from build123d import *

# Parameters (mm, degrees)
SKETCH1_W             = 254
SKETCH1_H             = 152.4
BOSS_EXTRUDE1_DEPTH   = 6
SKETCH2_W             = 25.4
SKETCH2_H             = 5.588
SKETCH2_W_2           = 31.75
SKETCH2_H_2           = 2.7432
TABS_TOP_BOTTOM_DEPTH = 6
SKETCH3_W             = 5.588
SKETCH3_H             = 25.4508
TABS_SIDE_DEPTH       = 6


with BuildPart() as part:
    # Sketch1 → Boss-Extrude1 (new body)
    with BuildSketch(Plane(origin=(0, 0, 0), x_dir=(1, 0, 0), z_dir=(0, 1, 0))):
        Rectangle(SKETCH1_W, SKETCH1_H)
    extrude(amount=BOSS_EXTRUDE1_DEPTH)

    # Sketch2 → Tabs - Top/Bottom (add)
    with BuildSketch(Plane(origin=(0, 6, 0), x_dir=(1, 0, 0), z_dir=(0, 1, 0))):
        with Locations((95.25, 78.994)):
            Rectangle(SKETCH2_W, SKETCH2_H)
        with Locations((-95.25, 78.994)):
            Rectangle(SKETCH2_W, SKETCH2_H)
        with Locations((-31.75, 78.994)):
            Rectangle(SKETCH2_W, SKETCH2_H)
        with Locations((31.75, 78.994)):
            Rectangle(SKETCH2_W, SKETCH2_H)
        with Locations((-95.25, -77.5716)):
            Rectangle(SKETCH2_W_2, SKETCH2_H_2)
        with Locations((0, -77.5716)):
            Rectangle(SKETCH2_W_2, SKETCH2_H_2)
        with Locations((95.25, -77.5716)):
            Rectangle(SKETCH2_W_2, SKETCH2_H_2)
    extrude(amount=-TABS_TOP_BOTTOM_DEPTH)

    # Sketch3 → Tabs - Side (add)
    with BuildSketch(Plane(origin=(0, 6, 0), x_dir=(1, 0, 0), z_dir=(0, 1, 0))):
        with Locations((-129.794, -38.1)):
            Rectangle(SKETCH3_W, SKETCH3_H)
        with Locations((-129.794, 0)):
            Rectangle(SKETCH3_W, SKETCH3_H)
        with Locations((-129.794, 38.1)):
            Rectangle(SKETCH3_W, SKETCH3_H)
        with Locations((129.794, -38.1)):
            Rectangle(SKETCH3_W, SKETCH3_H)
        with Locations((129.794, 38.1)):
            Rectangle(SKETCH3_W, SKETCH3_H)
        with Locations((129.794, 0)):
            Rectangle(SKETCH3_W, SKETCH3_H)
    extrude(amount=-TABS_SIDE_DEPTH)


solid = part.part
Work out the finished part from the listing and answer in its coordinate system (mm). A direction names the side the tool comes from. Round coordinates to 2 decimals unless told otherwise and drop trailing zeros. Write each loop counter-clockwise with the first axis right and the second up, starting at its lowest first coordinate (ties: lowest second). Pieces come first, ordered by that corner, then holes. Notation, with made-up numbers: (-39.75, 85.5) -> (-9.75, 85.5) arc R20 ccw to (-9.75, 108.5) -> close; hole circle Ø1 at (58.25, -36.5). An arc over 180 degrees is marked (long way). Answer as CSV lines item,"result". Start each with the question number.
(1) The part is cut by section A-A, the plane x = -22. Give the vertices of the cut face in (y, z), then the cut area to 3 significant figures.
(2) Each of these flat-tipped pins is pushed along its axis until it touches: pin 1 (3 mm diameter, centred on y = 2, z = 78, fed in from +X) (3 decimals); pin 2 (3 mm diameter, centred on y = 2.5, z = -80, fed in from -X); pin 3 (3 mm diameter, centred on y = 2, z = -79.5, fed in from +X); pin 4 (6 mm diameter, centred on x = -91, z = 0.5, fed in from -Y). Where does it stop, or does it pass through?
(3) The part is cut by section B-B, the plane z = -54.5. Give the vertices of the cut face in (x, y).
(4) A tool of negligible diameter and unlimited length cuts with its end or side. For faces 1 (the flat face through (47, 3, 76.2)), 2 (the flat face through (-119, 3, 76.2)), 3 (the flat face through (-130, 3, 12.725)), from which of +Z, -Z, +X, -X, +Y, -Y can it reach the whole face along a straight path? Write none if from no direction.
(5) The mould has two halves that part along Z. Classify faces 4 (the flat face through (130, 3, 25.375)), 5 (the flat face through (0, 3, -76.2)), 6 (the flat face through (-44.45, 3, -79)): +Z half, -Z half, draft (parallel to the pull), parting line (faces both ways), or undercut.
(6) Find the intervals of material crossed by probe 1 along Z at (x, y) = (-119, 1.15); probe 2 along X at (y, z) = (5.6, 68); probe 3 along Z at (x, y) = (-1.5, 2.5), in increasing order.
Output values:
1,outline,"(0, -81.79) -> (6, -81.79) -> (6, 76.2) -> (0, 76.2) -> close"
1,area,"948 mm²"
2,pin 1,"stops at x = 111.125"
2,pin 2,"stops at x = -107.95"
2,pin 3,"stops at x = 107.95"
2,pin 4,"stops at y = 0"
3,outline,"(-127, 0) -> (127, 0) -> (127, 6) -> (-127, 6) -> close"
4,face 1,"+Z, +Y, -Y"
4,face 2,"+Z, -X, +Y, -Y"
4,face 3,"-X, +Y, -Y"
5,face 4,"undercut"
5,face 5,"-Z half"
5,face 6,"draft"
6,probe 1,"z = -76.2 to 76.2"
6,probe 2,"x = -127 to 127"
6,probe 3,"z = -76.2 to 78.94"
